The model under review builds one solid part; all positions refer to its coordinate system, in mm. A direction names the side the tool comes from. Round coordinates to 2 decimals unless told otherwise and drop trailing zeros. Loops run counter-clockwise (first coordinate to the right, second up) from the corner with the lowest first, then second, coordinate; pieces in that order, holes last. Notation, with made-up numbers: (14.5, 79) -> (41.5, 79) arc R33 cw to (41.5, 107) -> close; hole circle Ø7 at (-4, 21.25). An arc over 180 degrees is marked (long way). Use CSV: the item, a comma, the result in double quotes. Start each with the question number.
```python
from build123d import *

# Parameters (mm, degrees)
SKETCH_1_R      = 1.25
SKETCH_1_R_2    = 3
SKETCH_1_W      = 6
SKETCH_1_H      = 6
EXTRUDE_1_DEPTH = 1
SKETCH_1_3_W    = 6
SKETCH_1_3_H    = 6
EXTRUDE_2_DEPTH = 4
EXTRUDE_START   = 4
SKETCH_1_4_R    = 3
SKETCH_1_4_R_2  = 0.675
EXTRUDE_5_DEPTH = 0.2


with BuildPart() as part:
    # Sketch 1 → Extrude 1 (new body)
    with BuildSketch(Plane(origin=(0, 0, 0), x_dir=(1, 0, 0), z_dir=(0, 1, 0))):
        with BuildLine():
            Line((-5.75, 3.5), (5.75, 3.5))
            ThreePointArc((5.75, 3.5), (8.224873734, 4.525126266), (9.25, 7))
            Line((9.25, 7), (9.25, 9.5))
            Line((9.25, 9.5), (21.5, 9.5))
            Line((21.5, 9.5), (27.5, 6.5))
            Line((27.5, 6.5), (27.5, 4.9))
            ThreePointArc((27.5, 4.9), (25.268114575, 2), (27.5, -0.9))
            Line((27.5, -0.9), (27.5, -6.5))
            Line((27.5, -6.5), (21.5, -9.5))
            Line((21.5, -9.5), (-21.5, -9.5))
            Line((-21.5, -9.5), (-27.5, -6.5))
            Line((-27.5, -6.5), (-27.5, -4.9))
            ThreePointArc((-27.5, -4.9), (-25.268114575, -2), (-27.5, 0.9))
            Line((-27.5, 0.9), (-27.5, 6.5))
            Line((-27.5, 6.5), (-21.5, 9.5))
            Line((-21.5, 9.5), (-9.25, 9.5))
            Line((-9.25, 9.5), (-9.25, 7))
            ThreePointArc((-9.25, 7), (-8.224873734, 4.525126266), (-5.75, 3.5))
        make_face()
        with Locations((-24.699999952, -5.700000209)):
            Circle(SKETCH_1_R, mode=Mode.SUBTRACT)
        with Locations((24.7, 5.7)):
            Circle(SKETCH_1_R, mode=Mode.SUBTRACT)
        with Locations((-17.5, 0)):
            Circle(SKETCH_1_R_2, mode=Mode.SUBTRACT)
        with Locations((-17.5, 0)):
            Rectangle(SKETCH_1_W, SKETCH_1_H)
    extrude(amount=EXTRUDE_1_DEPTH)

    # Sketch 1_3 → Extrude 2 (add)
    with BuildSketch(Plane(origin=(0, 0, 0), x_dir=(1, 0, 0), z_dir=(0, 1, 0))):
        with Locations((-17.5, 0)):
            Rectangle(SKETCH_1_3_W, SKETCH_1_3_H)
    extrude(amount=EXTRUDE_2_DEPTH)

    # Sketch 1_4 → Extrude 5 (add)
    with BuildSketch(Plane(origin=(0, 0, 0), x_dir=(1, 0, 0), z_dir=(0, 1, 0)).offset(EXTRUDE_START)):
        with Locations((-17.5, 0)):
            Circle(SKETCH_1_4_R)
        with Locations((-17.5, 0)):
            Circle(SKETCH_1_4_R_2, mode=Mode.SUBTRACT)
    extrude(amount=EXTRUDE_5_DEPTH)


solid = part.part
```
1. For faces 1 (the face through (-18, 2, 3)), 2 (the face through (-18, 2, -3)), 3 (the face through (-0.1, 0.5, -3.5)), 4 (the face through (-20.5, 2, 0)), list the 3-axis set-ups (+Z, -Z, +X, -X, +Y, -Y) from which the entire face can be reached by the end or side of a thin tool; tool diameter is ignored.
2. For line 1 along Y through (x, z) = (1.5, 8.5); line 2 along Z through (x, y) = (-20, 3.8); line 3 along X through (y, z) = (2.25, 0.5), list the stretches that pass through material, from the lowest coordinate up. Write a range as from..to.
3. Clearance check with flat-ended pins moving along their axes: P1, Ø2.5, axis at x = -16.5, y = 2.5, coming from the +Z side; P2, Ø0.8, axis at y = 0.5, z = -9, coming from the +X side; P3, Ø0.9, axis at y = 2.5, z = -0.5, coming from the -X side. State where each tip first meets the part, or that it passes through.
4. Take a section at B-B, the plane z = -5.7. Give the boundary of the cut face in (x, y), then the cut area to 3 significant figures.
5. Take a section at C-C, the plane z = -2.5. Give the boundary of the cut face in (x, y).
6. Take a section at D-D, the plane y = 2.3. Give the boundary of the cut face in (x, z), then the cut area to 3 significant figures.
7. Take a section at A-A, the plane z = 5.7. Give the boundary of the cut face in (x, y), then the cut area to 3 significant figures.
Results:
1,face 1,"+Z, +X, -X, +Y"
1,face 2,"-Z, +X, -X, +Y"
1,face 3,"-Z, +Y, -Y"
1,face 4,"+Z, -Z, -X, +Y"
2,line 1,"0..1"
2,line 2,"-3..3"
2,line 3,"-20.5..-14.5"
3,P1,"z = 3"
3,P2,"x = 23.3"
3,P3,"x = -20.5"
4,outline,"(-27.5, 0) -> (-9, 0) -> (-9, 1) -> (-27.5, 1) -> close; (9, 0) -> (23.45, 0) -> (23.45, 1) -> (9, 1) -> close; (25.95, 0) -> (27.5, 0) -> (27.5, 1) -> (25.95, 1) -> close"
4,area,"34.5 mm²"
5,outline,"(-27.5, 0) -> (25.31, 0) -> (25.31, 1) -> (-14.5, 1) -> (-14.5, 4) -> (-15.84, 4) -> (-15.84, 4.2) -> (-19.16, 4.2) -> (-19.16, 4) -> (-20.5, 4) -> (-20.5, 1) -> (-27.5, 1) -> close"
6,outline,"(-20.5, -3) -> (-14.5, -3) -> (-14.5, 3) -> (-20.5, 3) -> close"
6,area,"36.0 mm²"
7,outline,"(-27.5, 0) -> (-25.95, 0) -> (-25.95, 1) -> (-27.5, 1) -> close; (-23.45, 0) -> (27.5, 0) -> (27.5, 1) -> (-23.45, 1) -> close"
7,area,"52.5 mm²"
